Answer from the drawing. Dimensions are ordinates in mm from the lowest x, y and z of the part. A direction names the side the tool comes from. Coordinates: 2 decimals unless noted, no trailing zeros. Order: outer loops, then holes, each group sorted by start corner. A loop starts at its lowest first (then second) coordinate and runs counter-clockwise, first axis right, second up. Notation, with made-up numbers: (77, 14) - (110, 14) arc R26 cw to (110, 52) - close; hole circle Ø8 at (71, 26). An arc over 180 degrees is marked (long way). Use a Markdown table: item, result. Add a question column.
Item 1: For the marked faces 1 and 2, determine the directions among +Z, -Z, +X, -X, +Y, -Y from which every point of the face is accessible in a straight line to the end or side of a thin tool.
Item 2: Find the intervals of material crossed by line 1 along X through (y, z) = (70, 98); line 2 along Y through (x, z) = (52.5, 15), in increasing order.
Item 3: The part is cut by section B-B, the plane y = 7. Give the vertices of the cut face in (x, z), then the cut area to 3 significant figures.
Item 4: The part is cut by section C-C, the plane x = 56.5. Give the vertices of the cut face in (y, z), then the cut area to 3 significant figures.
Item 5: The mould has two halves that part along X. Classify the marked faces 3, 4 and 5: released by +X, released by -X, zero draft, split by the parting line, or undercut.
Item 6: The part is cut by section A-A, the plane z = 31.5. Give the vertices of the cut face in (x, y) (1 decimal).
Item 7: A flat-ended cylindrical pin translates along its axis: P1, Ø10, axis at x = 30, z = 67, coming from the +Y side. Find the tip coordinate at first contact, or state that the pin passes through.
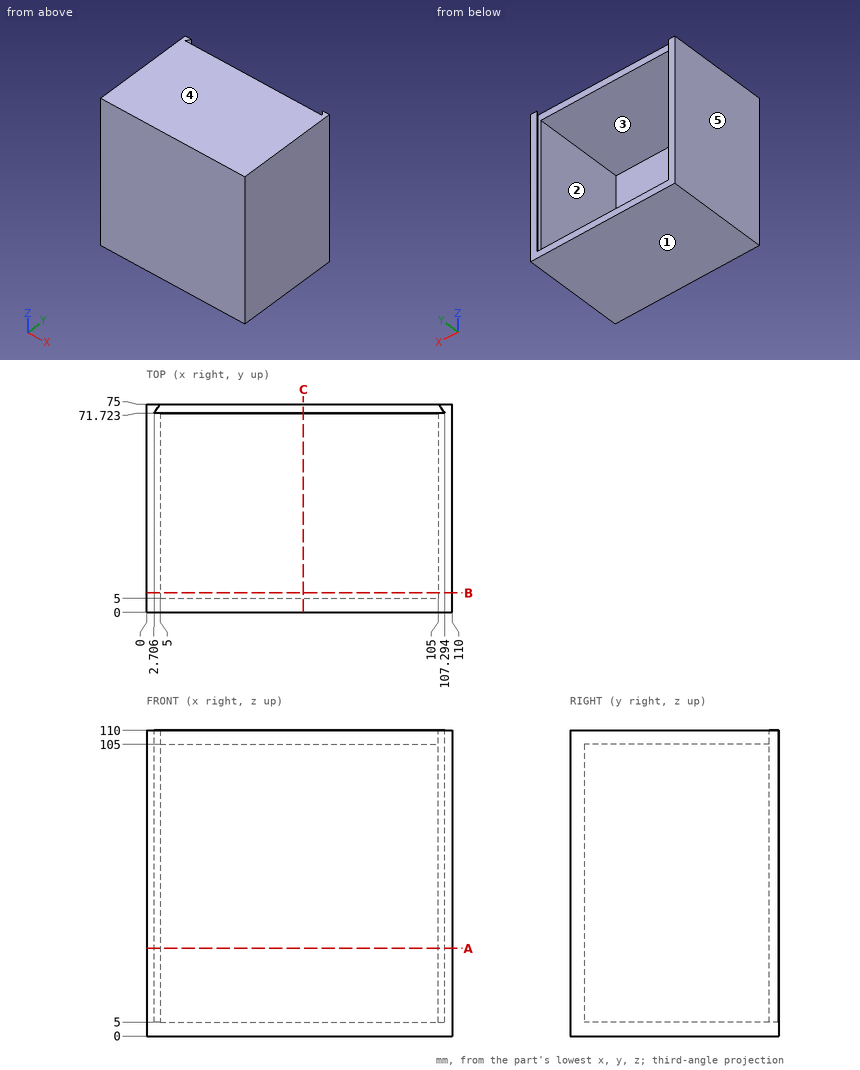
Solution:
| question | item | result |
|---|---|---|
| 1 | face 1 | -Z, +X, -X, +Y, -Y |
| 1 | face 2 | +Y |
| 2 | line 1 | x = 0 to 5, 105 to 110 |
| 2 | line 2 | y = 0 to 5 |
| 3 | outline | (0, 0) - (110, 0) - (110, 110) - (0, 110) - close; hole (5, 5) - (105, 5) - (105, 105) - (5, 105) - close |
| 3 | area | 2,100 mm2 |
| 4 | outline | (0, 0) - (75, 0) - (75, 5) - (5, 5) - (5, 105) - (71.72, 105) - (71.72, 110) - (0, 110) - close |
| 4 | area | 1,230 mm2 |
| 5 | face 3 | undercut |
| 5 | face 4 | zero draft |
| 5 | face 5 | released by -X |
| 6 | outline | (0, 0) - (110, 0) - (110, 75) - (105, 75) - (107.3, 71.7) - (105, 71.7) - (105, 5) - (5, 5) - (5, 71.7) - (2.7, 71.7) - (5, 75) - (0, 75) - close |
| 7 | P1 | stops at y = 5 |
